Verification items for the finished model (mm, model axes). Face numbers are marked on the shaded views. Round coordinates to 2 decimals unless told otherwise and drop trailing zeros. Order: outer loops, then holes, each group sorted by start corner. A loop starts at its lowest first (then second) coordinate and runs counter-clockwise, first axis right, second up.
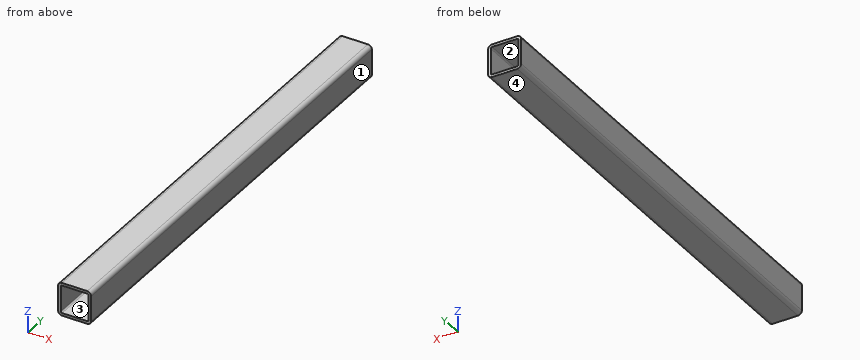
Autodesk Inventor part; units mm, degrees
ref_plane "YZ Plane" through (0, 0, 0) normal (1, 0, 0) x (0, 1, 0)
ref_plane "XZ Plane" through (0, 0, 0) normal (0, 1, 0) x (-1, 0, 0)
ref_plane "XY Plane" through (0, 0, 0) normal (0, 0, 1) x (1, 0, 0)
sketch "Sketch1" plane through (0, 0, 0) normal (0, 1, 0) x (-1, 0, 0)
  line L0 (-9.5, 11.5) -> (9.5, 11.5) construction
  line L1 (11.5, 9.5) -> (11.5, -9.5) construction
  line L2 (9.5, -11.5) -> (-9.5, -11.5) construction
  line L3 (-11.5, -9.5) -> (-11.5, 9.5) construction
  line L4 (-11.5, 11.5) -> (11.5, -11.5) construction
  line L5 (11.5, 11.5) -> (-11.5, -11.5) construction
  arc A0 (11.5, 9.5) -> (9.5, 11.5) centre (9.5, 9.5) ccw construction
  arc A1 (9.5, -11.5) -> (11.5, -9.5) centre (9.5, -9.5) ccw construction
  arc A2 (-11.5, -9.5) -> (-9.5, -11.5) centre (-9.5, -9.5) ccw construction
  arc A3 (-9.5, 11.5) -> (-11.5, 9.5) centre (-9.5, 9.5) ccw construction
  line L6 (-9.5, -12.5) -> (9.5, -12.5)
  arc A4 (9.5, -12.5) -> (12.5, -9.5) centre (9.5, -9.5) ccw
  line L7 (12.5, -9.5) -> (12.5, 9.5)
  arc A5 (12.5, 9.5) -> (9.5, 12.5) centre (9.5, 9.5) ccw
  line L8 (9.5, 12.5) -> (-9.5, 12.5)
  arc A6 (-9.5, 12.5) -> (-12.5, 9.5) centre (-9.5, 9.5) ccw
  line L9 (-12.5, 9.5) -> (-12.5, -9.5)
  arc A7 (-12.5, -9.5) -> (-9.5, -12.5) centre (-9.5, -9.5) ccw
  line L10 (10.5, -9.5) -> (10.5, 9.5)
  arc A8 (10.5, 9.5) -> (9.5, 10.5) centre (9.5, 9.5) ccw
  line L11 (9.5, 10.5) -> (-9.5, 10.5)
  arc A9 (-9.5, 10.5) -> (-10.5, 9.5) centre (-9.5, 9.5) ccw
  line L12 (-10.5, 9.5) -> (-10.5, -9.5)
  arc A10 (-10.5, -9.5) -> (-9.5, -10.5) centre (-9.5, -9.5) ccw
  line L13 (-9.5, -10.5) -> (9.5, -10.5)
  arc A11 (9.5, -10.5) -> (10.5, -9.5) centre (9.5, -9.5) ccw
  point P0 (0, 0)
  point P1 (0, 0)
  point P2 (0, 0)
  dimension "d10" = 2
  dimension "depth" = 25
  dimension "width" = 25
  dimension "thickness" = 2
extrude "Extrusion1" add sketch "Sketch1" along normal blind 350
equation "\"d10\" = thickness"
properties part number "beam 25x25x2 1-2" material "Steel"
1) Sectioned sample at B-B on z = 1.25. Record the cut outline in (x, y), then the cut area to 3 significant figures.
2) Sectioned sample at C-C on y = 251. Record the cut outline in (x, z), then the cut area to 3 significant figures.
3) Sectioned sample at A-A on x = 1.75. Record the cut outline in (y, z), then the cut area to 3 significant figures.
4) Scan lines: probe 1 along X at (y, z) = (223, 9); probe 2 along X at (y, z) = (242, 10). Record each from-to range of solid material in increasing order.
5) Draft check along X on the marked faces 1, 2, 3 and 4. Enter one of: released by +X, released by -X, zero draft, split by the parting line, or undercut.
Returned:
1. outline: (-12.5, 0) - (-10.5, 0) - (-10.5, 350) - (-12.5, 350) - close; (10.5, 0) - (12.5, 0) - (12.5, 350) - (10.5, 350) - close
1. area: 1,400 mm2
2. outline: (-12.5, -9.5) arc R3 ccw to (-9.5, -12.5) - (9.5, -12.5) arc R3 ccw to (12.5, -9.5) - (12.5, 9.5) arc R3 ccw to (9.5, 12.5) - (-9.5, 12.5) arc R3 ccw to (-12.5, 9.5) - close; hole (-10.5, -9.5) arc R1 ccw to (-9.5, -10.5) - (9.5, -10.5) arc R1 ccw to (10.5, -9.5) - (10.5, 9.5) arc R1 ccw to (9.5, 10.5) - (-9.5, 10.5) arc R1 ccw to (-10.5, 9.5) - close
2. area: 177 mm2
3. outline: (0, -12.5) - (350, -12.5) - (350, -10.5) - (0, -10.5) - close; (0, 10.5) - (350, 10.5) - (350, 12.5) - (0, 12.5) - close
3. area: 1,400 mm2
4. probe 1: x = -12.5 to -10.5, 10.5 to 12.5
4. probe 2: x = -12.46 to -10.37, 10.37 to 12.46
5. face 1: released by +X
5. face 2: undercut
5. face 3: undercut
5. face 4: zero draft
